```python
from build123d import *

# Parameters (mm, degrees)
SKETCH1_W                                       = 200
SKETCH1_H                                       = 100
BOSS_EXTRUDE1_DEPTH                             = 12
F_9_0_9_DIAMETER_HOLE1_D                        = 9
CBORE_FOR_M5_SOCKET_HEAD_CAP_SCREW1_D           = 6
CBORE_FOR_M5_SOCKET_HEAD_CAP_SCREW1_CBORE_D     = 11
CBORE_FOR_M5_SOCKET_HEAD_CAP_SCREW1_CBORE_DEPTH = 8
CHAMFER1_SIZE                                   = 8


with BuildPart() as part:
    # Sketch1 → Boss-Extrude1 (new body)
    with BuildSketch(Plane(origin=(0, 0, 0), x_dir=(1, 0, 0), z_dir=(0, 1, 0))):
        with Locations((-100, 0)):
            Rectangle(SKETCH1_W, SKETCH1_H)
    extrude(amount=BOSS_EXTRUDE1_DEPTH)

    # Ø9.0 (9) Diameter Hole1 (through all)
    with Locations(Plane(origin=(0, 12, 0), x_dir=(-1, 0, 0), z_dir=(0, 1, 0))):
        with Locations((185, 30), (15, 30), (15, -30), (185, -30)):
            Hole(F_9_0_9_DIAMETER_HOLE1_D / 2)

    # CBORE for M5 Socket Head Cap Screw1 (through all)
    with Locations(Plane.XZ):
        with Locations((-150, 39), (-50, 39), (-150, -39), (-50, -39)):
            CounterBoreHole(CBORE_FOR_M5_SOCKET_HEAD_CAP_SCREW1_D / 2, CBORE_FOR_M5_SOCKET_HEAD_CAP_SCREW1_CBORE_D / 2, CBORE_FOR_M5_SOCKET_HEAD_CAP_SCREW1_CBORE_DEPTH)

    # Chamfer1
    chamfer1_edges = [part.edges().sort_by_distance(p)[0] for p in [
        (-200, 6, -50),
        (0, 6, -50),
        (0, 6, 50),
        (-200, 6, 50),
    ]]
    chamfer(chamfer1_edges, length=CHAMFER1_SIZE)


solid = part.part
```
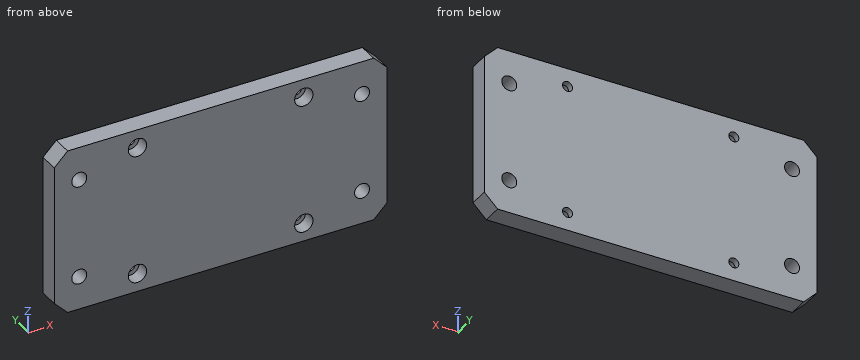
Check sheet for the modelled part. Datum: model origin and axes. Units: mm. Round coordinates to 2 decimals unless told otherwise and drop trailing zeros. Loops run counter-clockwise (first coordinate to the right, second up) from the corner with the lowest first, then second, coordinate; pieces in that order, holes last. Notation, with made-up numbers: M -15,37.5 L 32,37.5 A22 ccw 32,52.5 Z; hole C 13,-14.5 d10. An arc over 180 degrees is marked long. Answer as a JSON object with one key per item and string values.
1. Gauge pin test, flat ends, axial feed: P1, Ø5.5, axis at x = -185, z = -30, coming from the -Y side; P2, Ø3.5, axis at x = -147.5, z = 37.5, coming from the -Y side. Record the tip position at first contact, or that the pin passes through.
Reply:
{"P1": "passes through", "P2": "stops at y = 8"}
2. Section check A-A (x = -185). Record the boundary of the cut face in (y, z), plus the area to 3 significant figures.
Reply:
{"outline": "M 0,-50 L 12,-50 L 12,-34.5 L 0,-34.5 Z; M 0,-25.5 L 12,-25.5 L 12,25.5 L 0,25.5 Z; M 0,34.5 L 12,34.5 L 12,50 L 0,50 Z", "area": "984 mm²"}
3. Scan lines: line 1 (Z direction, x = -185, y = 3); line 2 (Z direction, x = -150, y = 9.75); line 3 (X direction, y = 3.25, z = 38). Record each from-to range of solid material in increasing order.
Reply:
{"line 1": "z = -50 to -34.5, -25.5 to 25.5, 34.5 to 50", "line 2": "z = -50 to -42, -36 to 36, 42 to 50", "line 3": "x = -200 to -155.41, -144.59 to -55.41, -44.59 to 0"}
4. Section check B-B (y = 5). State how many separate pieces and enclosed holes the cut face has, plus the area to 3 significant figures.
Reply:
{"separate pieces": "1", "enclosed holes": "8", "area": "19,200 mm²"}
5. Section check D-D (z = -39). Record the boundary of the cut face in (x, y).
Reply:
{"outline": "M -200,0 L -155.5,0 L -155.5,8 L -153,8 L -153,12 L -200,12 Z; M -147,8 L -144.5,8 L -144.5,0 L -55.5,0 L -55.5,8 L -53,8 L -53,12 L -147,12 Z; M -47,8 L -44.5,8 L -44.5,0 L 0,0 L 0,12 L -47,12 Z"}
6. Section check C-C (z = 30). Record the boundary of the cut face in (x, y), plus the area to 3 significant figures.
Reply:
{"outline": "M -200,0 L -189.5,0 L -189.5,12 L -200,12 Z; M -180.5,0 L -19.5,0 L -19.5,12 L -180.5,12 Z; M -10.5,0 L 0,0 L 0,12 L -10.5,12 Z", "area": "2,180 mm²"}
